Verification items for the finished model (mm, model axes). Round coordinates to 2 decimals unless told otherwise and drop trailing zeros. Loops run counter-clockwise (first coordinate to the right, second up) from the corner with the lowest first, then second, coordinate; pieces in that order, holes last.
from build123d import *

# Parameters (mm, degrees)
BOSS_EXTRUDE2_DEPTH     = 304.8
F_1_4_CLEARANCE_HOLE2_D = 6.7564


with BuildPart() as part:
    # Sketch1 → Boss-Extrude2 (new body)
    with BuildSketch(Plane.XY):
        with BuildLine():
            Line((-1.143, -8.256814656), (-1.143, 12.7))
            Line((-1.143, 12.7), (1.143, 12.7))
            Line((1.143, 12.7), (1.143, -12.7))
            ThreePointArc((1.143, -12.7), (0.537985791, -10.201615922), (-1.143, -8.256814656))
        make_face()
    extrude(amount=BOSS_EXTRUDE2_DEPTH)

    # 1/4 Clearance Hole2 (through all)
    with Locations(Plane.ZY.offset(1.143)):
        with Locations((9.050000188, 0), (295.749999812, 0)):
            Hole(F_1_4_CLEARANCE_HOLE2_D / 2)


solid = part.part
1. Section check A-A (y = 0). Enter the section's corners in (x, z).
2. Release check for a two-part mould opening along Y. For faces 1 (the face through (-1.143, 2, 150)), 2 (the face through (0.016, 0.149, 12.425)), 3 (the face through (0.016, 0.149, 299.125)) record: released by +Y, released by -Y, zero draft, split by the parting line, or undercut.
3. Section check C-C (x = -0.1). Enter the section's corners in (y, z), then the cut area to 3 significant figures.
4. Section check B-B (z = 295.75). Enter the section's corners in (x, y).
5. Section check D-D (z = 65). Enter the section's corners in (x, y).
6. Scan lines: L1, parallel to Z at x = 0, y = -1; L2, parallel to Z at x = 0.05, y = -2; L3, parallel to Y at x = 0.55, z = 295.75. Record each from-to range of solid material in increasing order.
Taken from the geometry:
1. outline: (-1.14, 0) - (1.14, 0) - (1.14, 5.67) - (-1.14, 5.67) - close; (-1.14, 12.43) - (1.14, 12.43) - (1.14, 292.37) - (-1.14, 292.37) - close; (-1.14, 299.13) - (1.14, 299.13) - (1.14, 304.8) - (-1.14, 304.8) - close
2. face 1: zero draft
2. face 2: undercut
2. face 3: undercut
3. outline: (-9.23, 0) - (12.7, 0) - (12.7, 304.8) - (-9.23, 304.8) - close; hole circle Ø6.76 at (0, 9.05); hole circle Ø6.76 at (0, 295.75)
3. area: 6,610 mm2
4. outline: (-1.14, -8.26) arc R5.46 cw to (1.14, -12.7) - (1.14, -3.38) - (-1.14, -3.38) - close; (-1.14, 3.38) - (1.14, 3.38) - (1.14, 12.7) - (-1.14, 12.7) - close
5. outline: (-1.14, -8.26) arc R5.46 cw to (1.14, -12.7) - (1.14, 12.7) - (-1.14, 12.7) - close
6. L1: z = 0 to 5.82, 12.28 to 292.52, 298.98 to 304.8
6. L2: z = 0 to 6.33, 11.77 to 293.03, 298.47 to 304.8
6. L3: y = -10.23 to -3.38, 3.38 to 12.7
